Source: CAD feature listing. Evaluate the final solid. Frame: model axes, mm. A direction names the side the tool comes from. Round coordinates to 2 decimals unless told otherwise and drop trailing zeros. Loops run counter-clockwise (first coordinate to the right, second up) from the corner with the lowest first, then second, coordinate; pieces in that order, holes last. Notation, with made-up numbers: (-10.5, 28) -> (46.5, 28) arc R18 ccw to (46.5, 54) -> close; hole circle Ø7 at (7, 36). An arc over 180 degrees is marked (long way). Put each result on its own line as item: value. Start each with the question number.
1. Contact query for flat-ended pins moving along their axis: pin 1 (3 mm diameter, centred on x = 0.5, z = 8.5, fed in from -Y); pin 2 (1.8 mm diameter, centred on x = -11.5, y = 2.5, fed in from -Z); pin 3 (1 mm diameter, centred on x = -2.5, z = 3, fed in from -Y). Output: stop coordinate, or through.
2. Draft query along Y for faces 6 (the flat face through (10, -12.43, 1)), 7 (the flat face through (-9.031, 4, 1)), 8 (the cylindrical face through (-2.9, 1.34, 9.63)). Return one class per face: pulls with the +Y half, pulls with the -Y half, needs draft (parallel to the pull), parting line crosses it, or undercut.
3. Set-up query: faces 1 (the flat face through (2.5, -7.653, 5.5)), 2 (the flat face through (10, -17, 2.2)), 3 (the flat face through (-2.3, -5, 1)), 4 (the flat face through (-10.8, 4.2, 5.9)), 5 (the flat face through (-8.211, -5, 4)). Return all of +Z, -Z, +X, -X, +Y, -Y with unobstructed straight access to the full face (end or side cutting, diameter ignored); none if empty.
4. Material intervals for L1, parallel to X at y = 3, z = 3; L2, parallel to X at y = -1.25, z = 0.75; L3, parallel to Y at x = 12, z = 5.75, sorted ascending.
5. Cut plane B-B (x = 0). Return the cut outline in (y, z), then the cut area to 3 significant figures.
6. Cut plane A-A (y = -1.75). State how many separate pieces and enclosed holes the cut face has, then the cut area to 3 significant figures.
```python
from build123d import *

# Parameters (mm, degrees)
EXTRUDE_1_DEPTH      = 8.4
SKETCH_2_W           = 3.875941336
SKETCH_2_H           = 10.635716013
CUT_EXTRUDE_1_DEPTH  = 150
SKETCH_3_W           = 2
SKETCH_3_H           = 5.614214587
CUT_EXTRUDE_2_DEPTH  = 2.5
SKETCH_4_W           = 7.533258122
SKETCH_4_H           = 2.2
CUT_EXTRUDE_3_DEPTH  = 2.45
SKETCH_5_W           = 2
SKETCH_5_H           = 5.614214587
CUT_EXTRUDE_4_DEPTH  = 2.5
SKETCH_6_W           = 2.766629061
SKETCH_6_H           = 2.133374911
CUT_EXTRUDE_5_DEPTH  = 2.45
SKETCH_7_W           = 16.422219314
SKETCH_7_H           = 5.5
CUT_EXTRUDE_6_DEPTH  = 10
SKETCH_8_R           = 0.45
EXTRUDE_2_DEPTH      = 8
SKETCH_9_R           = 1.1
SKETCH_9_R_2         = 0.75
SKETCH_9_W           = 1
SKETCH_9_H           = 0.97451262
CUT_EXTRUDE_7_DEPTH  = 10
SKETCH_10_W          = 16.251149316
SKETCH_10_H          = 2
CUT_EXTRUDE_8_DEPTH  = 2.5
CUT_EXTRUDE_9_DEPTH  = 2.5
SKETCH_12_W          = 4.6
SKETCH_12_H          = 9.297061896
CUT_EXTRUDE_10_DEPTH = 1.45
CHAMFER_1_SIZE       = 2
CUT_EXTRUDE_11_DEPTH = 0.2
SKETCH_14_R          = 0.45
EXTRUDE_3_DEPTH      = 2.5


with BuildPart() as part:
    # Эскиз1 → Вытянуть1 (new body)
    with BuildSketch(Plane.XY):
        with BuildLine():
            Line((-9.125, -11.858221261), (-8.211109657, -9.652950274))
            Line((-8.211109657, -9.652950274), (8.211109657, -9.652950274))
            Line((8.211109657, -9.652950274), (9.125, -11.858221261))
            Line((9.125, -11.858221261), (9.125, -18.516991449))
            Line((9.125, -18.516991449), (7.754731336, -17.684929687))
            ThreePointArc((7.754731336, -17.684929687), (7.527121952, -17.698805472), (7.460452641, -17.916873745))
            Line((7.460452641, -17.916873745), (8.074001716, -19.832909478))
            ThreePointArc((8.074001716, -19.832909478), (8.282801368, -20.196609982), (8.622375639, -20.442708876))
            Line((8.622375639, -20.442708876), (9.699802329, -20.918536331))
            ThreePointArc((9.699802329, -20.918536331), (10.213465399, -20.997740615), (10.697503229, -20.808451293))
            Line((10.697503229, -20.808451293), (10.834983302, -20.707015208))
            Line((10.834983302, -20.707015208), (9.939315034, -20.125628034))
            Line((9.939315034, -20.125628034), (11.669448618, -12.430286305))
            Line((11.669448618, -12.430286305), (14.148872473, -6.816071718))
            Line((14.148872473, -6.816071718), (14.148872473, 4.381463669))
            ThreePointArc((14.148872473, 4.381463669), (13.855979254, 5.08857045), (13.148872473, 5.381463669))
            Line((13.148872473, 5.381463669), (-13.148872473, 5.381463669))
            ThreePointArc((-13.148872473, 5.381463669), (-13.855979254, 5.08857045), (-14.148872473, 4.381463669))
            Line((-14.148872473, 4.381463669), (-14.148872473, -6.816071718))
            Line((-14.148872473, -6.816071718), (-11.669448618, -12.430286305))
            Line((-11.669448618, -12.430286305), (-9.939315034, -20.125628034))
            Line((-9.939315034, -20.125628034), (-10.834983302, -20.707015208))
            Line((-10.834983302, -20.707015208), (-10.697503229, -20.808451293))
            ThreePointArc((-10.697503229, -20.808451293), (-10.213465399, -20.997740615), (-9.699802329, -20.918536331))
            Line((-9.699802329, -20.918536331), (-8.622375639, -20.442708876))
            ThreePointArc((-8.622375639, -20.442708876), (-8.282801368, -20.196609982), (-8.074001716, -19.832909478))
            Line((-8.074001716, -19.832909478), (-7.460452641, -17.916873745))
            ThreePointArc((-7.460452641, -17.916873745), (-7.527121952, -17.698805472), (-7.754731336, -17.684929687))
            Line((-7.754731336, -17.684929687), (-9.125, -18.516991449))
            Line((-9.125, -18.516991449), (-9.125, -11.858221261))
        make_face()
    extrude(amount=EXTRUDE_1_DEPTH)

    # Эскиз2 → Вырез-Вытянуть1 (cut)
    with BuildSketch(Plane(origin=(14.148872473, 0, 0), x_dir=(0, 0, -1), z_dir=(1, 0, 0))):
        with Locations((-8.137970668, -17.748144312)):
            Rectangle(SKETCH_2_W, SKETCH_2_H)
        with Locations((-0.262029332, -17.748144312)):
            Rectangle(SKETCH_2_W, SKETCH_2_H)
    extrude(amount=-CUT_EXTRUDE_1_DEPTH, mode=Mode.SUBTRACT)

    # Эскиз3 → Вырез-Вытянуть2 (cut)
    with BuildSketch(Plane(origin=(14.148872473, 0, 0), x_dir=(0, 0, -1), z_dir=(1, 0, 0))):
        with Locations((-4.2, -9.623179012)):
            Rectangle(SKETCH_3_W, SKETCH_3_H)
    extrude(amount=-CUT_EXTRUDE_2_DEPTH, mode=Mode.SUBTRACT)

    # Эскиз4 → Вырез-Вытянуть3 (cut)
    with BuildSketch(Plane(origin=(14.148872473, 0, 0), x_dir=(0, 0, -1), z_dir=(1, 0, 0))):
        with Locations((-4.2, -11.330286305)):
            Rectangle(SKETCH_4_W, SKETCH_4_H)
    extrude(amount=-CUT_EXTRUDE_3_DEPTH, mode=Mode.SUBTRACT)

    # Эскиз5 → Вырез-Вытянуть4 (cut)
    with BuildSketch(Plane.ZY.offset(14.148872473)):
        with Locations((4.2, -9.623179012)):
            Rectangle(SKETCH_5_W, SKETCH_5_H)
    extrude(amount=-CUT_EXTRUDE_4_DEPTH, mode=Mode.SUBTRACT)

    # Эскиз6 → Вырез-Вытянуть5 (cut)
    with BuildSketch(Plane.ZY.offset(14.148872473)):
        with Locations((6.583314531, -11.296973761)):
            Rectangle(SKETCH_6_W, SKETCH_6_H)
        with Locations((1.81668547, -11.296973761)):
            Rectangle(SKETCH_6_W, SKETCH_6_H)
    extrude(amount=-CUT_EXTRUDE_5_DEPTH, mode=Mode.SUBTRACT)

    # Эскиз7 → Вырез-Вытянуть6 (cut)
    with BuildSketch(Plane.XZ.offset(9.652950274)):
        with Locations((0, 4.2)):
            Rectangle(SKETCH_7_W, SKETCH_7_H)
    extrude(amount=-CUT_EXTRUDE_6_DEPTH, mode=Mode.SUBTRACT)

    # Эскиз8 → Вытянуть2 (add)
    with BuildSketch(Plane.XZ.offset(-0.347049726)):
        with Locations(Location((0, 2.93, 0), (0, 0, 90))):
            Circle(SKETCH_8_R)
        with Locations(Location((0, 5.47, 0), (0, 0, 90))):
            Circle(SKETCH_8_R)
        with Locations(Location((2.54, 5.47, 0), (0, 0, 90))):
            Circle(SKETCH_8_R)
        with Locations(Location((2.54, 2.93, 0), (0, 0, 90))):
            Circle(SKETCH_8_R)
        with Locations(Location((5.08, 5.47, 0), (0, 0, 90))):
            Circle(SKETCH_8_R)
        with Locations(Location((5.08, 2.93, 0), (0, 0, 90))):
            Circle(SKETCH_8_R)
        with Locations(Location((-2.54, 5.47, 0), (0, 0, 90))):
            Circle(SKETCH_8_R)
        with Locations(Location((-2.54, 2.93, 0), (0, 0, 90))):
            Circle(SKETCH_8_R)
        with Locations(Location((-5.08, 5.47, 0), (0, 0, 90))):
            Circle(SKETCH_8_R)
        with Locations(Location((-5.08, 2.93, 0), (0, 0, 90))):
            Circle(SKETCH_8_R)
    extrude(amount=EXTRUDE_2_DEPTH)

    # Эскиз9 → Вырез-Вытянуть7 (cut)
    with BuildSketch(Plane(origin=(0, 0, 0), x_dir=(-1, 0, 0), z_dir=(0, 0, -1))):
        with Locations((-10.785, 2.881463669)):
            Circle(SKETCH_9_R)
        with Locations((10.785, 2.881463669)):
            Circle(SKETCH_9_R)
        with Locations((-12, -5.867574023)):
            Circle(SKETCH_9_R_2)
        with Locations(Location((12, -5.867574023, 0), (0, 0, 180))):
            Circle(SKETCH_9_R_2)
        with Locations((4.770217249, -9.651420054)):
            Rectangle(SKETCH_9_W, SKETCH_9_H)
        with Locations((-4.770217249, -9.651420054)):
            Rectangle(SKETCH_9_W, SKETCH_9_H)
    extrude(amount=-CUT_EXTRUDE_7_DEPTH, mode=Mode.SUBTRACT)

    # Эскиз10 → Вырез-Вытянуть8 (cut)
    with BuildSketch(Plane(origin=(0, 0, 0), x_dir=(-1, 0, 0), z_dir=(0, 0, -1))):
        Polygon((-12.539432173, 3.987610768), (-12.539432173, 6.55660708), (-9.030567827, 6.55660708), (-9.030567827, 3.987610768), (-9.030567827, 1.868541782), (-10.785, 0.855619895), (-12.539432173, 1.868541782), align=None)
        Polygon((9.030567827, 6.55660708), (9.030567827, 3.987610768), (9.030567827, 1.868541782), (10.785, 0.855619895), (12.539432173, 1.868541782), (12.539432173, 3.987610768), (12.539432173, 6.55660708), align=None)
        with Locations((0, 2.868541782)):
            Rectangle(SKETCH_10_W, SKETCH_10_H)
    extrude(amount=-CUT_EXTRUDE_8_DEPTH, mode=Mode.SUBTRACT)

    # Эскиз11 → Вырез-Вытянуть9 (cut)
    with BuildSketch(Plane.XY.offset(8.4)):
        Polygon((12.539432173, 1.868541782), (12.539432173, 5.381463669), (9.030567827, 5.381463669), (9.030567827, 1.868541782), (10.785, 0.855619895), align=None)
        Polygon((-9.030567827, 5.381463669), (-12.539432173, 5.381463669), (-12.539432173, 1.868541782), (-10.785, 0.855619895), (-9.030567827, 1.868541782), align=None)
    extrude(amount=-CUT_EXTRUDE_9_DEPTH, mode=Mode.SUBTRACT)

    # Эскиз12 → Вырез-Вытянуть10 (cut)
    with BuildSketch(Plane(origin=(0, 0, 0), x_dir=(-1, 0, 0), z_dir=(0, 0, -1))):
        with Locations((0, -6.301481222)):
            Rectangle(SKETCH_12_W, SKETCH_12_H)
    extrude(amount=-CUT_EXTRUDE_10_DEPTH, mode=Mode.SUBTRACT)

    # Фаска1
    # the kernel refuses this chamfer: 2 mm, written as the material it takes off along each edge
    with BuildSketch(Plane(origin=(-2.3, -1.652950274, 0), x_dir=(0, 0.9996219169112968, -0.027495876610586365), z_dir=(1, 0, 0))) as chamfer_1_piece_1:
        Polygon((CHAMFER_1_SIZE * 0.999621916911, CHAMFER_1_SIZE * 0.0274958766106), (-CHAMFER_1_SIZE * 0.0274958766106, CHAMFER_1_SIZE * 0.999621916911), (0, 0), align=None)
    extrude(amount=4.6, mode=Mode.SUBTRACT)

    # Эскиз13 → Вырез-Вытянуть11 (cut)
    with BuildSketch(Plane(origin=(0, 0, 0), x_dir=(-1, 0, 0), z_dir=(0, 0, -1))):
        Polygon((6.423321525, -9.652950274), (7.482877419, -9.652950274), (6.953099472, -8.645062752), align=None)
    extrude(amount=-CUT_EXTRUDE_11_DEPTH, mode=Mode.SUBTRACT)

    # Эскиз14 → Вытянуть3 (add)
    with BuildSketch(Plane.XY.offset(8.4)):
        with Locations((0, 4.151463669)):
            Circle(SKETCH_14_R)
        with Locations((0, 1.611463669)):
            Circle(SKETCH_14_R)
        with Locations((2.54, 4.151463669)):
            Circle(SKETCH_14_R)
        with Locations((2.54, 1.611463669)):
            Circle(SKETCH_14_R)
        with Locations((5.08, 4.151463669)):
            Circle(SKETCH_14_R)
        with Locations((5.08, 1.611463669)):
            Circle(SKETCH_14_R)
        with Locations((-2.54, 4.151463669)):
            Circle(SKETCH_14_R)
        with Locations((-2.54, 1.611463669)):
            Circle(SKETCH_14_R)
        with Locations((-5.08, 4.151463669)):
            Circle(SKETCH_14_R)
        with Locations((-5.08, 1.611463669)):
            Circle(SKETCH_14_R)
    extrude(amount=EXTRUDE_3_DEPTH)


solid = part.part
```
Solution:
1. pin 1: stops at y = -9.65
1. pin 2: stops at z = 2.5
1. pin 3: stops at y = -7.65
2. face 6: pulls with the -Y half
2. face 7: needs draft
2. face 8: undercut
3. face 1: -Y
3. face 2: -Z, +X, -X, -Y
3. face 3: -Z, -Y
3. face 4: +Z, +Y
3. face 5: none
4. L1: x = -14.15 to -11.88, -9.69 to 9.69, 11.88 to 14.15
4. L2: x = -14.15 to -2.3, 2.3 to 14.15
4. L3: y = -10.23 to -6.62, -5.12 to 5.38
5. outline: (-9.65, 6.95) -> (0.35, 6.95) -> (0.35, 5.92) -> (-7.65, 5.92) -> (-7.65, 5.02) -> (0.35, 5.02) -> (0.35, 3.38) -> (-7.65, 3.38) -> (-7.65, 2.48) -> (0.35, 2.48) -> (0.35, 1.45) -> (-1.1, 1.45) -> (0.35, 0) -> (1.87, 0) -> (1.87, 2.5) -> (3.87, 2.5) -> (3.87, 0) -> (5.38, 0) -> (5.38, 8.4) -> (4.6, 8.4) -> (4.6, 10.9) -> (3.7, 10.9) -> (3.7, 8.4) -> (2.06, 8.4) -> (2.06, 10.9) -> (1.16, 10.9) -> (1.16, 8.4) -> (-9.65, 8.4) -> close
5. area: 71.7 mm^2
6. separate pieces: 11
6. enclosed holes: 0
6. area: 147 mm^2
